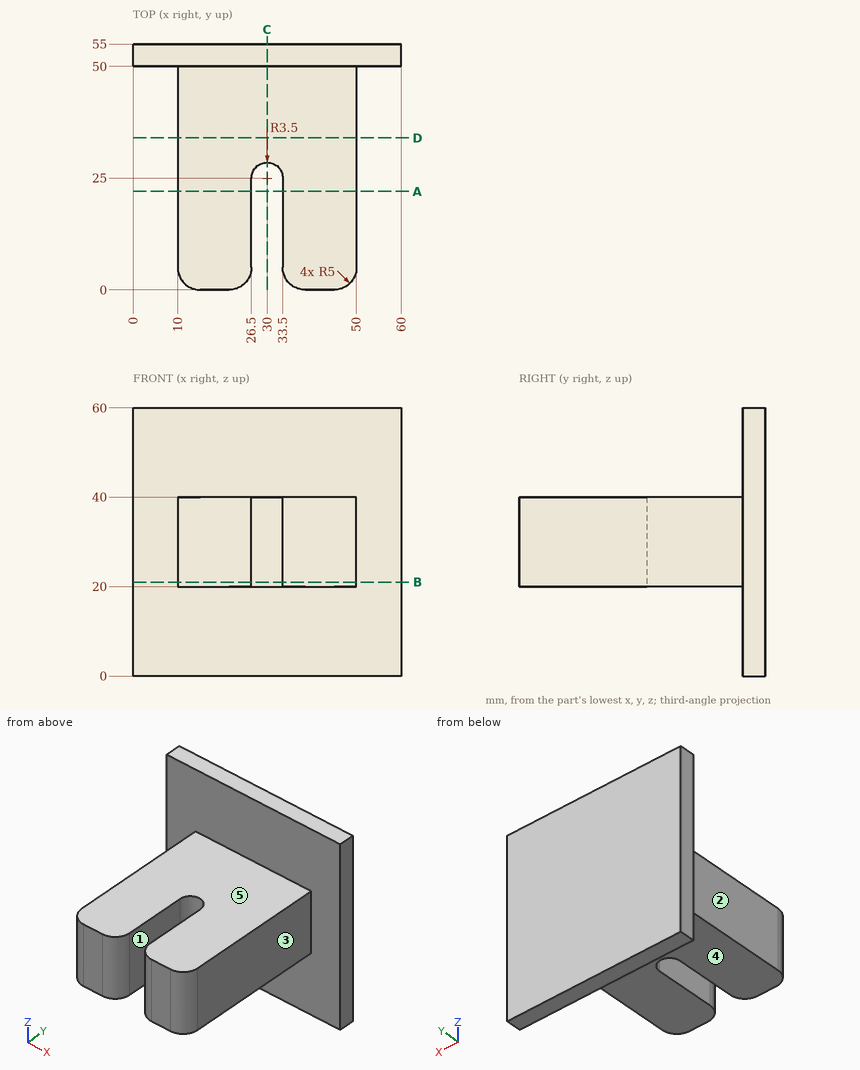
Job drawing, mm, ordinate dimensions from the low corner. One solid piece. A direction names the side the tool comes from. Round coordinates to 2 decimals unless told otherwise and drop trailing zeros. Loops run counter-clockwise (first coordinate to the right, second up) from the corner with the lowest first, then second, coordinate; pieces in that order, holes last.
Item 1: Cut at D-D, the plane y = 34. Give the cut face in (x, z).
Item 2: Drill centre lines: line 1 (X direction, y = 7.5, z = 21.5); line 2 (Y direction, x = 5, z = 50); line 3 (Z direction, x = 47, y = 44.5). Where is each one in solid material? Low to high.
Item 3: Cut at B-B, the plane z = 21. Give the cut face in (x, y), then the cut area to 3 significant figures.
Item 4: Cut at C-C, the plane x = 30. Give the cut face in (y, z), then the cut area to 3 significant figures.
Item 5: Drop flat-ended pins along their axis: P1, Ø6, axis at y = 15.5, z = 32.5, coming from the +X side; P2, Ø16, axis at y = 35, z = 32, coming from the -X side; P3, Ø5, axis at x = 11.5, y = 16, coming from the +Z side. Give the stop position or say it passes through.
Item 6: Cut at A-A, the plane y = 22. Give the cut face in (x, z).
Item 7: 3-axis set-ups, long thin cutter, end or side, ignore diameter. For the marked faces 1, 2, 3, 4 and 5: which of +Z, -Z, +X, -X, +Y, -Y reach the whole face in a straight line?
A:
1. outline: (10, 20) - (50, 20) - (50, 40) - (10, 40) - close
2. line 1: x = 10 to 26.5, 33.5 to 50
2. line 2: y = 50 to 55
2. line 3: z = 20 to 40
3. outline: (0, 50) - (10, 50) - (10, 5) arc R5 ccw to (15, 0) - (21.5, 0) arc R5 ccw to (26.5, 5) - (26.5, 25) arc R3.5 cw to (33.5, 25) - (33.5, 5) arc R5 ccw to (38.5, 0) - (45, 0) arc R5 ccw to (50, 5) - (50, 50) - (60, 50) - (60, 55) - (0, 55) - close
3. area: 2,080 mm2
4. outline: (28.5, 20) - (50, 20) - (50, 0) - (55, 0) - (55, 60) - (50, 60) - (50, 40) - (28.5, 40) - close
4. area: 730 mm2
5. P1: stops at x = 50
5. P2: stops at x = 10
5. P3: stops at z = 40
6. outline: (10, 20) - (26.5, 20) - (26.5, 40) - (10, 40) - close; (33.5, 20) - (50, 20) - (50, 40) - (33.5, 40) - close
7. face 1: +Z, -Z, -Y
7. face 2: +Z, -Z, -X, -Y
7. face 3: +Z, -Z, +X, -Y
7. face 4: -Z, +X, -X, -Y
7. face 5: +Z, +X, -X, -Y
